The model under review builds one solid part; all positions refer to its coordinate system, in mm. Face numbers are marked on the shaded views. A direction names the side the tool comes from. Give positions to 0.01 mm unless a question says otherwise; leave off trailing zeros. Write each loop counter-clockwise with the first axis right and the second up, starting at its lowest first coordinate (ties: lowest second). Pieces come first, ordered by that corner, then holes. Notation, with made-up numbers: (-6.5, 56.5) - (34.5, 56.5) arc R20 cw to (34.5, 80.5) - close; hole circle Ø1 at (53, 4.25). An arc over 180 degrees is marked (long way). Write item = value, one per line.
```python
from build123d import *

# Parameters (mm, degrees)
F0_R     = 15
F1_DEPTH = 112
F2_R     = 15
F2_R_2   = 7.5
F3_DEPTH = 102
F4_R     = 7.5
F4_R_2   = 5
F5_DEPTH = 62


with BuildPart() as f1:
    # F0 (on Front) → F1 (new body)
    with BuildSketch(Plane.XZ):
        Circle(F0_R)
    extrude(amount=F1_DEPTH)

    # F2 (on Front) → F3 (cut)
    with BuildSketch(Plane.XZ):
        Circle(F2_R)
        Circle(F2_R_2, mode=Mode.SUBTRACT)
    extrude(amount=F3_DEPTH, mode=Mode.SUBTRACT)

    # F4 (on face) → F5 (cut)
    with BuildSketch(Plane(origin=(0, 0, 0), x_dir=(-1, 0, 0), z_dir=(0, 1, 0))):
        Circle(F4_R)
        Circle(F4_R_2, mode=Mode.SUBTRACT)
    extrude(amount=-F5_DEPTH, mode=Mode.SUBTRACT)


solid = f1.part
```
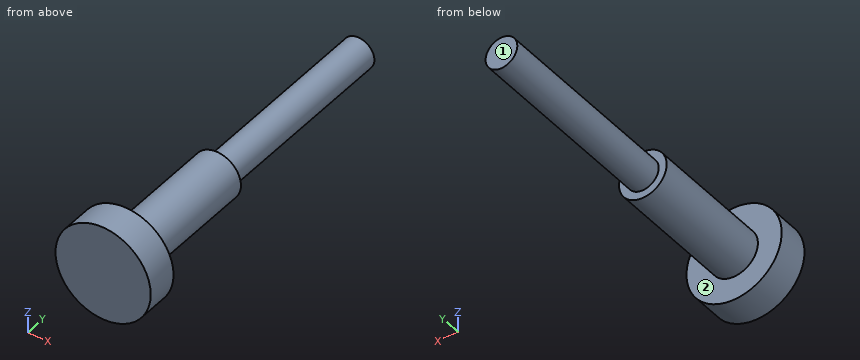
1. Take a section at A-A on z = 0. Give the boundary of the cut face in (x, y), and give its area (3 significant figures).
Findings below:
outline = (-15, -112) - (15, -112) - (15, -102) - (7.5, -102) - (7.5, -62) - (5, -62) - (5, 0) - (-5, 0) - (-5, -62) - (-7.5, -62) - (-7.5, -102) - (-15, -102) - close
area = 1,520 mm²
2. For line 1 (Y direction, x = 9.5, z = -4); line 2 (Y direction, x = -5.75, z = -3); line 3 (Z direction, x = -2.5, y = -87.5), list the stretches that pass through material, from the lowest coordinate up. Write a range as from..to.
Findings below:
line_1 = -112..-102
line_2 = -112..-62
line_3 = -7.07..7.07
3. Insertion check: P1, Ø12, axis at y = -42, z = -7, coming from the +X side; P2, Ø10, axis at x = -7.5, y = -34.5, coming from the +Z side; P3, Ø8, axis at x = -9, z = 4.5, coming from the +Y side. Each pin has a flat end and moves straight along its axis. Give the tip position at first contact, or say it passes through.
Findings below:
P1 = 4.9
P2 = 4.33
P3 = -62
4. Take a section at C-C on y = -96. Give the boundary of the cut face in (x, z), and give its area (3 significant figures).
Findings below:
outline = circle Ø15 at (0, 0)
area = 177 mm²
5. Take a section at D-D on z = 6. Give the boundary of the cut face in (x, y), and give its area (3 significant figures).
Findings below:
outline = (-13.75, -112) - (13.75, -112) - (13.75, -102) - (4.5, -102) - (4.5, -62) - (-4.5, -62) - (-4.5, -102) - (-13.75, -102) - close
area = 635 mm²
6. Take a section at B-B on x = 0. Give the boundary of the cut face in (y, z), and give its area (3 significant figures).
Findings below:
outline = (-112, -15) - (-102, -15) - (-102, -7.5) - (-62, -7.5) - (-62, -5) - (0, -5) - (0, 5) - (-62, 5) - (-62, 7.5) - (-102, 7.5) - (-102, 15) - (-112, 15) - close
area = 1,520 mm²
7. Machinability: for the marked faces 1 and 2, which of the approach directions +Z, -Z, +X, -X, +Y, -Y give a long, thin tool a straight path to every point of the face, cutting with its end or side? Answer none if there is none.
Findings below:
face_1 = +Z, -Z, +X, -X, +Y
face_2 = +Y
